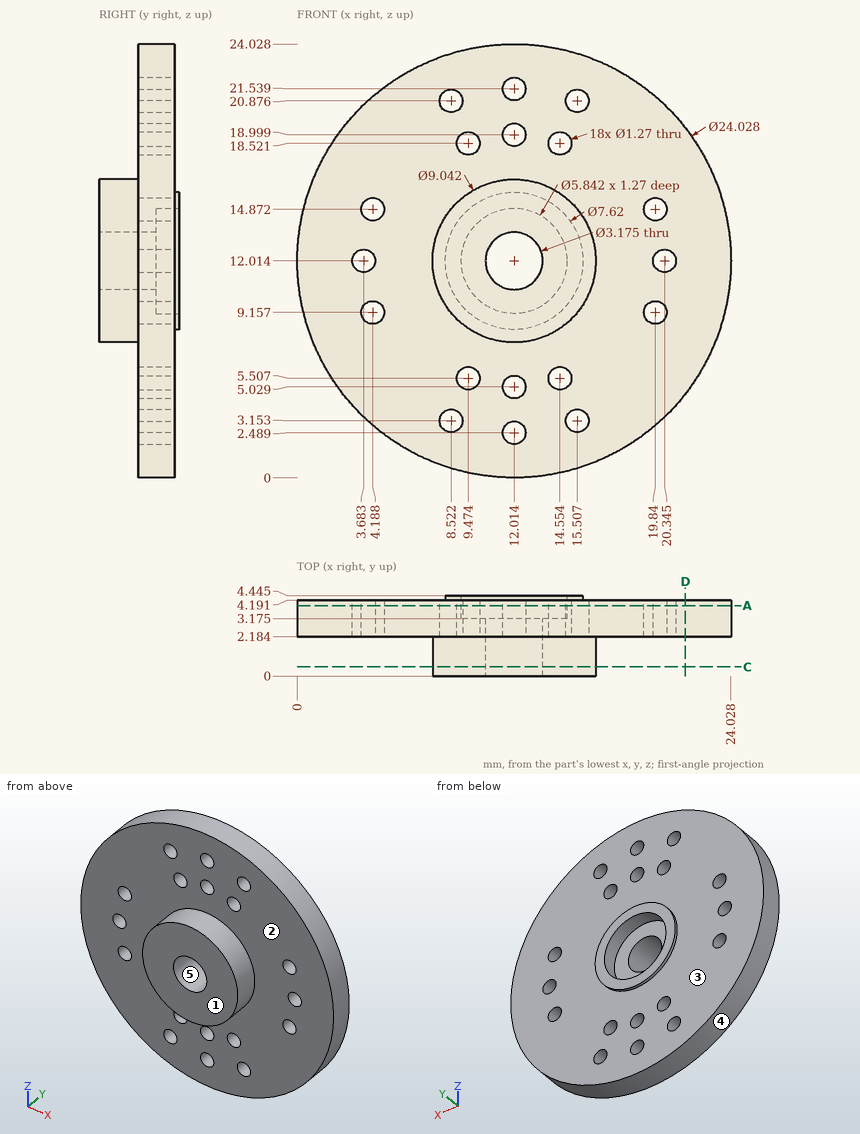
Job drawing, mm, ordinate dimensions from the low corner. One solid piece. A direction names the side the tool comes from. Give positions to 0.01 mm unless a question says otherwise; leave off trailing zeros. Loops run counter-clockwise (first coordinate to the right, second up) from the corner with the lowest first, then second, coordinate; pieces in that order, holes last. Notation, with made-up numbers: (11, 54.5) - (25, 54.5) arc R12 ccw to (25, 69.5) - close; hole circle Ø10 at (-28, 7). An arc over 180 degrees is marked (long way). Use one line per item in the form item = value.
(1) Cut at A-A (y = 3.9). Count the separate pieces of the cut face and the enclosed holes in it, then the cut area to 3 significant figures.
Determined:
separate_pieces = 1
enclosed_holes = 19
area = 404 mm^2
(2) Pull direction Z, two halves, no side cores. Call the marked faces 3, 4 and 5: pulls with the +Z half, pulls with the -Z half, needs draft (parallel to the pull), parting line crosses it, or undercut.
Determined:
face_3 = needs draft
face_4 = parting line crosses it
face_5 = undercut
(3) Cut at C-C (y = 0.5). Give the cut face in (x, z) (1 decimal).
Determined:
outline = circle Ø9 at (12, 12); hole circle Ø3.2 at (12, 12)
(4) 3-axis set-ups, long thin cutter, end or side, ignore diameter. For the marked faces 1 and 2: which of +Z, -Z, +X, -X, +Y, -Y reach the whole face in a straight line?
Determined:
face_1 = +Z, -Z, +X, -X, -Y
face_2 = -Y
(5) Cut at D-D (x = 21.5). Give the cut face in (y, z) (1 decimal).
Determined:
outline = (2.2, 4.6) - (4.2, 4.6) - (4.2, 19.4) - (2.2, 19.4) - close
(6) Drop flat-ended pins along their axis: P1, Ø2, axis at x = 4.19, z = 14.87, coming from the -Y side; P2, Ø3, axis at x = 11, z = 12.5, coming from the +Y side (3 decimals); P3, Ø1.5, axis at x = 15.51, z = 20.88, coming from the +Y side; P4, Ø1.9, axis at x = 12.01, z = 12.01, coming from the +Y side. Give the stop position or say it passes through.
Determined:
P1 = 2.18
P2 = 3.175
P3 = 4.19
P4 = through
(7) Drill centre lines: L1, parallel to Y at x = 16.25, z = 22.5 (1 decimal); L2, parallel to X at y = 2.1, z = 12.25 (1 decimal); L3, parallel to X at y = 1.4, z = 11.25 (1 decimal). Where is each one in solid material? Low to high.
Determined:
L1 = 2.2 to 4.2
L2 = 7.5 to 10.4, 13.6 to 16.5
L3 = 7.6 to 10.6, 13.4 to 16.5
